Could you check a few things on this model? Use its own coordinates, in mm. A direction names the side the tool comes from. Coordinates: 2 decimals unless noted, no trailing zeros. Write each loop counter-clockwise with the first axis right and the second up, starting at its lowest first coordinate (ties: lowest second). Pieces come first, ordered by that corner, then holes.
Item 1: I want a section at B-B on x = 25.4. Please give me the cut outline in (y, z).
Item 2: I want a section at A-A on z = 12.7. Please give me the cut outline in (x, y) (3 decimals), then the cut area to 3 significant figures.
Item 3: I want a section at D-D on y = -48.5. Please give me the cut outline in (x, z).
Item 4: I want a section at C-C on y = -76.2. Please give me the cut outline in (x, z) (3 decimals).
Item 5: Which directions (+Z, -Z, +X, -X, +Y, -Y) give clear straight access to the entire face, cutting with the end or side of a thin tool? Please do faces 1 (the flat face through (63.5, -44, 60)), 2 (the flat face through (35, -44, 57.15)).
Item 6: For P1, Ø7.5, axis at x = 11.13, y = -11.13, coming from the -Z side; P2, Ø8, axis at y = -34, z = 15.5, coming from the +X side, each with a flat end and sliding along its axis, tell me the tip position at first contact or that it passes through.
Item 7: Thinking about a two-plate mould opening in Y: for faces 3 (the cylindrical face through (22.37, -10.17, 60.28)), 4 (the flat face through (6.35, -44, 28)), 5 (the flat face through (3.13, -86.32, 2.5)), which applies, +Y half, -Y half, draft (parallel to the pull), parting line (faces both ways), or undercut?
Item 8: If I drill on probe 1 along Y at (x, z) = (25, 60); probe 2 along Y at (x, z) = (25.4, 58.75); probe 3 along Z at (x, y) = (25, -26), over which ranges is the centre line in solid material (lowest first)?
from build123d import *

# Parameters (mm, degrees)
F1_DEPTH = 88.9
F3_D     = 6.35
F4_SIZE  = 5.08
F6_D     = 6.35


with BuildPart() as f1:
    # F0 (on Front) → F1 (new body)
    with BuildSketch(Plane.XZ):
        Polygon((0, 63.5), (0, 0), (6.35, 0), (6.35, 57.15), (63.5, 57.15), (63.5, 63.5), align=None)
    extrude(amount=F1_DEPTH)

    # F3 (through all)
    with Locations(Plane.YZ.offset(6.35)):
        with Locations((-76.2, 12.7), (-12.7, 12.7)):
            Hole(F3_D / 2)

    # F4
    f4_edges = [f1.edges().sort_by_distance(p)[0] for p in [
        (3.175, -88.9, 0),
        (3.175, 0, 0),
        (63.5, -88.9, 60.325),
        (63.5, 0, 60.325),
    ]]
    chamfer(f4_edges, length=F4_SIZE)

    # F6 (through all)
    with Locations(Plane.XY.offset(63.5)):
        with Locations((25.4, -11.1252), (11.1252, -11.1252), (11.1252, -77.8002), (25.4, -77.8002)):
            Hole(F6_D / 2)


solid = f1.part
Response values:
1. outline: (-88.9, 57.15) - (-80.98, 57.15) - (-80.98, 63.5) - (-88.9, 63.5) - close; (-74.63, 57.15) - (-14.3, 57.15) - (-14.3, 63.5) - (-74.63, 63.5) - close; (-7.95, 57.15) - (0, 57.15) - (0, 63.5) - (-7.95, 63.5) - close
2. outline: (0, -88.9) - (6.35, -88.9) - (6.35, -79.375) - (0, -79.375) - close; (0, -73.025) - (6.35, -73.025) - (6.35, -15.875) - (0, -15.875) - close; (0, -9.525) - (6.35, -9.525) - (6.35, 0) - (0, 0) - close
2. area: 484 mm2
3. outline: (0, 0) - (6.35, 0) - (6.35, 57.15) - (63.5, 57.15) - (63.5, 63.5) - (0, 63.5) - close
4. outline: (0, 0) - (6.35, 0) - (6.35, 9.525) - (0, 9.525) - close; (0, 15.875) - (6.35, 15.875) - (6.35, 57.15) - (8.383, 57.15) - (8.383, 63.5) - (0, 63.5) - close; (13.867, 57.15) - (22.658, 57.15) - (22.658, 63.5) - (13.867, 63.5) - close; (28.142, 57.15) - (63.5, 57.15) - (63.5, 63.5) - (28.142, 63.5) - close
5. face 1: +Z, -Z, +X, +Y, -Y
5. face 2: -Z, +X, +Y, -Y
6. P1: stops at z = 57.15
6. P2: stops at x = 6.35
7. face 3: undercut
7. face 4: draft
7. face 5: -Y half
8. probe 1: y = -88.9 to -80.95, -74.65 to -14.27, -7.98 to 0
8. probe 2: y = -88.9 to -80.98, -74.63 to -14.3, -7.95 to 0
8. probe 3: z = 57.15 to 63.5
